Check sheet for the modelled part. Datum: model origin and axes. Units: mm. A direction names the side the tool comes from. Round coordinates to 2 decimals unless told otherwise and drop trailing zeros. Write each loop counter-clockwise with the first axis right and the second up, starting at its lowest first coordinate (ties: lowest second). Pieces come first, ordered by that corner, then holes. Notation, with made-up numbers: (-17.75, -11) -> (37.25, -11) arc R33 cw to (37.25, 24) -> close; hole circle Ø8 at (13, 37.5). An arc over 180 degrees is marked (long way). One line per item, written item: value. Start each with the question number.
```python
from build123d import *

# Parameters (mm, degrees)
F1_DEPTH = 30
F3_DEPTH = 50


with BuildPart() as f1:
    # F0 (on Front) → F1 (new body)
    with BuildSketch(Plane.XZ):
        Polygon((-3, 0), (0, 0), (3, 0), (3, 15), (13.842538, 31.805932), (7.842538, 31.805932), (0, 19.649999), (-7.842538, 31.805932), (-13.842538, 31.805932), (-3, 15), align=None)
    extrude(amount=F1_DEPTH)

    # F2 (on Right) → F3 (cut, symmetric)
    with BuildSketch(Plane.YZ):
        Polygon((-23.980264, 0), (0, 0), (-23.980264, 12.434211), align=None)
        Polygon((-23.980264, 20.131581), (0, 32.269739), (-23.980264, 32.269739), align=None)
        Polygon((0, 5.729885), (0, 25.460526), (-19.255204, 15.714065), align=None)
    extrude(amount=F3_DEPTH, both=True, mode=Mode.SUBTRACT)


solid = f1.part
```
1. Cross-section at A-A (x = -10.75). Record the cut outline in (y, z).
2. Material ranges on probe 1 along X at (y, z) = (-19.5, 13); probe 2 along Y at (x, z) = (4, 21); probe 3 along X at (y, z) = (-25, 20.5), recorded low to high.
3. Cross-section at D-D (y = -13). Record the cut outline in (x, z).
4. Cross-section at C-C (y = -10). Record the cut outline in (x, z).
5. Cross-section at B-B (z = 10.5). Record the cut outline in (x, y).
6. Release check for a two-part mould opening along Y. For faces 1 (the face through (-7, -23.98, 26)), 2 (the face through (9, 0, 29)), 3 (the face through (7, -23.98, 26)), 4 (the face through (10.9, -0.5, 31.806)) record: +Y half, -Y half, draft (parallel to the pull), parting line (faces both ways), or undercut.
7. Access from +Z, -Z, +X, -X, +Y, -Y to the whole of each face (thin tool, end or side, straight path). Record for faces 5 (the face through (-2.03, -9.493, 20.656)), 6 (the face through (-7.171, -12.61, 25.887)), 7 (the face through (0, -23.98, 6)), 8 (the face through (3, -18, 11)).
8. Depth check by flat-ended pin: pin 1 Ø1.5 at (y, z) = (-5, 23.5) entering from +X; pin 2 Ø1.5 at (x, y) = (6.5, -7) entering from +Z; pin 3 Ø7.5 at (y, z) = (-17.5, 8) entering from +X. Enter the tip coordinate at first touch or a pass-through.
Working result:
1. outline: (-30, 27.01) -> (-23.98, 27.01) -> (-23.98, 31.81) -> (-30, 31.81) -> close; (-10.39, 27.01) -> (0, 27.01) -> (0, 31.81) -> (-0.92, 31.81) -> close
2. probe 1: x = -3 to 3
2. probe 2: y = -30 to -23.98, -22.26 to -8.81
2. probe 3: x = -6.55 to -0.55, 0.55 to 6.55
3. outline: (-9.9, 25.69) -> (-5.5, 18.88) -> (5.5, 18.88) -> (9.9, 25.69) -> (3.9, 25.69) -> (0, 19.65) -> (-3.9, 25.69) -> close; (-3, 6.74) -> (3, 6.74) -> (3, 12.47) -> (-3, 12.47) -> close
4. outline: (-10.88, 27.21) -> (-6.48, 20.4) -> (-0.48, 20.4) -> (-4.88, 27.21) -> close; (-3, 5.19) -> (3, 5.19) -> (3, 10.92) -> (-3, 10.92) -> close; (0.48, 20.4) -> (6.48, 20.4) -> (10.88, 27.21) -> (4.88, 27.21) -> close
5. outline: (-3, -30) -> (3, -30) -> (3, -23.98) -> (-3, -23.98) -> close; (-3, -20.25) -> (3, -20.25) -> (3, -9.2) -> (-3, -9.2) -> close
6. face 1: undercut
6. face 2: +Y half
6. face 3: undercut
6. face 4: draft
7. face 5: +X, -X, +Y
7. face 6: +Z, +X, -X
7. face 7: -Z, +X, -X
7. face 8: -Z, +X, +Y, -Y
8. pin 1: stops at x = 8.97
8. pin 2: stops at z = 29.11
8. pin 3: stops at x = 3
